```python
from build123d import *

# Parameters (mm, degrees)
BOSS_EXTRUDE1_DEPTH  = 83.0326
SKETCH6_W            = 61.8998
SKETCH6_H            = 21.463
BOSS_EXTRUDE3_DEPTH  = 3.175
SKETCH7_W            = 16.5354
SKETCH7_H            = 9.525
CUT_EXTRUDE2_DEPTH   = 91.420129415
SKETCH8_W            = 5.08
SKETCH8_H            = 25.4
CUT_EXTRUDE3_DEPTH   = 108.64212172
SKETCH15_W           = 27.7241
SKETCH15_H           = 45.085
BOSS_EXTRUDE5_DEPTH  = 3.175
SKETCH21_W           = 1.651
SKETCH21_H           = 45.085
BOSS_EXTRUDE10_DEPTH = 16.9926
SKETCH22_W           = 20.1676
SKETCH22_H           = 45.085
BOSS_EXTRUDE11_DEPTH = 1.5875
SKETCH23_W           = 29.3116
SKETCH23_H           = 45.085
BOSS_EXTRUDE12_DEPTH = 1.5875
SKETCH24_W           = 21.7551
SKETCH24_H           = 6.35
BOSS_EXTRUDE13_DEPTH = 1.5875
SKETCH25_W           = 61.8998
SKETCH25_H           = 25.4
CUT_EXTRUDE4_DEPTH   = 3.175


with BuildPart() as part:
    # Sketch1 → Boss-Extrude1 (new body)
    with BuildSketch(Plane(origin=(0, 0, 0), x_dir=(1, 0, 0), z_dir=(0, 1, 0))):
        Polygon((-30.9499, -3.477149156), (30.9499, -3.477149156), (30.9499, 17.985850844), (24.0411, 17.985850844), (24.0411, 14.810850844), (27.7749, 14.810850844), (27.7749, 5.285850844), (-27.7749, 5.285850844), (-27.7749, 14.810850844), (-24.0411, 14.810850844), (-24.0411, 17.985850844), (-30.9499, 17.985850844), align=None)
    extrude(amount=BOSS_EXTRUDE1_DEPTH)

    # Sketch6 → Boss-Extrude3 (add)
    with BuildSketch(Plane(origin=(0, 83.0326, 0), x_dir=(1, 0, 0), z_dir=(0, 1, 0))):
        with Locations((0, 7.254350844)):
            Rectangle(SKETCH6_W, SKETCH6_H)
    extrude(amount=BOSS_EXTRUDE3_DEPTH)

    # Sketch7 → Cut-Extrude2 (cut, through all)
    with BuildSketch(Plane.XZ.offset(-83.0326)):
        with Locations((0, -10.048350844)):
            Rectangle(SKETCH7_W, SKETCH7_H)
    extrude(amount=-CUT_EXTRUDE2_DEPTH, mode=Mode.SUBTRACT)

    # Sketch8 → Cut-Extrude3 (cut, through all)
    with BuildSketch(Plane.ZY.offset(30.9499)):
        with Locations((-0.274453158, 60.28364576)):
            Rectangle(SKETCH8_W, SKETCH8_H)
        with Locations((-0.274453158, 25.92395424)):
            Rectangle(SKETCH8_W, SKETCH8_H)
    extrude(amount=-CUT_EXTRUDE3_DEPTH, mode=Mode.SUBTRACT)

    # Sketch15 → Boss-Extrude5 (add)
    with BuildSketch(Plane.ZY.offset(30.9499)):
        with Locations((-19.676493716, 22.5425)):
            Rectangle(SKETCH15_W, SKETCH15_H)
    extrude(amount=BOSS_EXTRUDE5_DEPTH)

    # Sketch21 → Boss-Extrude10 (add)
    with BuildSketch(Plane.ZY.offset(34.1249)):
        with Locations((-6.639943716, 22.5425)):
            Rectangle(SKETCH21_W, SKETCH21_H)
    extrude(amount=BOSS_EXTRUDE10_DEPTH)

    # Sketch22 → Boss-Extrude11 (add)
    with BuildSketch(Plane(origin=(0, 0, -33.538543716), x_dir=(-1, 0, 0), z_dir=(0, 0, -1))):
        with Locations((41.0337, 22.5425)):
            Rectangle(SKETCH22_W, SKETCH22_H)
    extrude(amount=BOSS_EXTRUDE11_DEPTH)

    # Sketch23 → Boss-Extrude12 (add)
    with BuildSketch(Plane.ZY.offset(51.1175)):
        with Locations((-20.470243716, 22.5425)):
            Rectangle(SKETCH23_W, SKETCH23_H)
    extrude(amount=BOSS_EXTRUDE12_DEPTH)

    # Sketch24 → Boss-Extrude13 (add)
    with BuildSketch(Plane(origin=(0, 45.085, 0), x_dir=(1, 0, 0), z_dir=(0, 1, 0))):
        with Locations((-41.82745, 20.470243716)):
            Rectangle(SKETCH24_W, SKETCH24_H)
    extrude(amount=BOSS_EXTRUDE13_DEPTH)

    # Sketch25 → Cut-Extrude4 (cut)
    with BuildSketch(Plane(origin=(0, 0, -17.985850844), x_dir=(-1, 0, 0), z_dir=(0, 0, -1))):
        with Locations((0, 12.7)):
            Rectangle(SKETCH25_W, SKETCH25_H)
    extrude(amount=-CUT_EXTRUDE4_DEPTH, mode=Mode.SUBTRACT)


solid = part.part
```
Design review of the part built by this model. Coordinates are the model's own, in mm. A direction names the side the tool comes from. Coordinates: 2 decimals unless noted, no trailing zeros. Write each loop counter-clockwise with the first axis right and the second up, starting at its lowest first coordinate (ties: lowest second). Pieces come first, ordered by that corner, then holes.
1) Add section A-A (y = 18.5). Write out the cut boundary in (x, z) (1 decimal).
2) Mouldability with a two-part tool opening along X and no side actions: class faces 1 (the flat face through (0, 26, -2.814)), 2 (the flat face through (-26, 54, -14.811)), 3 (the flat face through (30.95, 43, -7)) as +X half, -X half, draft (parallel to the pull), parting line (faces both ways), or undercut.
3) Machinability: for faces 4 (the flat face through (0, 47.584, 0)), 5 (the flat face through (28, 25.4, -16)), 6 (the flat face through (-43, 23, -33.539)), 7 (the flat face through (26, 54, -14.811)), which of the approach directions +Z, -Z, +X, -X, +Y, -Y give a long, thin tool a straight path to every point of the face, cutting with its end or side? Answer none if there is none.
4) Insertion check: pin 1 (16.5 mm diameter, centred on x = -13, y = 51.5, fed in from -Z); pin 2 (3.5 mm diameter, centred on x = 27, z = -16.5, fed in from -Y); pin 3 (8 mm diameter, centred on y = 14.5, z = -20.5, fed in from +X). Each pin has a flat end and moves straight along its axis. Give the tip position at first contact, or say it passes through.
5) To check wall thickness, follow L1, parallel to Y at x = -26.5, z = -1; L2, parallel to X at y = 5, z = -11 (1 decimal); L3, parallel to X at y = 75, z = -14. State the ranges of each line that lie inside material, in increasing order.
6) Add section C-C (z = -1). Write out the cut boundary in (x, y), plus the area to 3 significant figures.
7) Add section B-B (z = -26.5). Write out the cut boundary in (x, y) (1 decimal).
8) Add section D-D (x = -15.5). Write out the cut boundary in (y, z).
Check result:
1. outline: (-52.7, -35.1) - (-30.9, -35.1) - (-30.9, -14.8) - (-27.8, -14.8) - (-27.8, -5.3) - (27.8, -5.3) - (27.8, -14.8) - (30.9, -14.8) - (30.9, -2.8) - (-30.9, -2.8) - (-30.9, -5.8) - (-52.7, -5.8) - close; (-30.9, 2.3) - (30.9, 2.3) - (30.9, 3.5) - (-30.9, 3.5) - close; hole (-51.1, -33.5) - (-34.1, -33.5) - (-34.1, -7.5) - (-51.1, -7.5) - close
2. face 1: draft
2. face 2: undercut
2. face 3: +X half
3. face 4: +X, -X
3. face 5: -Z, +X, -Y
3. face 6: +Y, -Y
3. face 7: -Y
4. pin 1: stops at z = -5.29
4. pin 2: stops at y = 25.4
4. pin 3: stops at x = -30.95
5. L1: y = 0 to 13.22, 38.62 to 47.58, 72.98 to 86.21
5. L2: x = -52.7 to -51.1, -34.1 to -27.8, 27.8 to 30.9
5. L3: x = -30.95 to -27.77, 27.77 to 30.95
6. outline: (-30.95, 0) - (30.95, 0) - (30.95, 13.22) - (-30.95, 13.22) - close; (-30.95, 38.62) - (30.95, 38.62) - (30.95, 47.58) - (-30.95, 47.58) - close; (-30.95, 72.98) - (30.95, 72.98) - (30.95, 86.21) - (-30.95, 86.21) - close
6. area: 2,190 mm2
7. outline: (-52.7, 0) - (-51.1, 0) - (-51.1, 45.1) - (-52.7, 45.1) - close; (-34.1, 0) - (-30.9, 0) - (-30.9, 45.1) - (-34.1, 45.1) - close
8. outline: (0, -5.29) - (83.03, -5.29) - (83.03, -17.99) - (86.21, -17.99) - (86.21, 3.48) - (0, 3.48) - close; hole (13.22, -2.81) - (38.62, -2.81) - (38.62, 2.27) - (13.22, 2.27) - close; hole (47.58, -2.81) - (72.98, -2.81) - (72.98, 2.27) - (47.58, 2.27) - close
